Part model, mm, in its own coordinate system. Coordinates: 2 decimals unless noted, no trailing zeros. Loops run counter-clockwise (first coordinate to the right, second up) from the corner with the lowest first, then second, coordinate; pieces in that order, holes last. Notation, with made-up numbers: (33.5, 73) - (91.5, 73) arc R5 ccw to (91.5, 82) - close; hole circle Ø9 at (18, 17). An arc over 180 degrees is marked (long way). Use a Markdown table: item, result. Add a question column.
1) Probe probe 1 along Z at (x, y) = (110, -2.5); probe 2 along Z at (x, y) = (25.4, -0.8); probe 3 along Z at (x, y) = (61, -2.2). List the from-to ranges inside material, lowest first. Write a range as [from, to].
2) Band-saw the part on C-C (x = 109). Give the cut face in (y, z) (3 decimals), plus the area to 3 significant figures.
3) Band-saw the part on B-B (y = -1.05). Give the number of separate pieces and of enclosed holes in the cut face, plus the area to 3 significant figures.
4) Pull direction Z, two halves, no side cores. Call faces 1 (the face through (141.064, -1.565, 99.69)), 2 (the face through (0, -2, 51)), 3 (the face through (87.24, -1.57, 96.22)): +Z half, -Z half, draft (parallel to the pull), parting line (faces both ways), or undercut.
5) Drop flat-ended pins along their axis: P1, Ø8.5, axis at x = 136.525, z = 38.1, coming from the +Y side; P2, Ø6.5, axis at x = 92.075, z = 76.2, coming from the -Y side. Give the stop position or say it passes through.
6) Band-saw the part on D-D (z = 38.1). Give the cut face in (x, y) (1 decimal), plus the area to 3 significant figures.
7) Band-saw the part on A-A (z = 88.9). Give the cut face in (x, y) (1 decimal).
from build123d import *

# Parameters (mm, degrees)
F0_R     = 3.2385
F0_R_2   = 2.54
F0_R_3   = 4.191
F0_R_4   = 14.2875
F0_R_5   = 4.7625
F1_DEPTH = 3.175


with BuildPart() as f1:
    # F0 (on Front) → F1 (new body)
    with BuildSketch(Plane.XZ):
        with BuildLine():
            ThreePointArc((0, 6.35), (1.859872, 1.859872), (6.35, 0))
            Line((6.35, 0), (136.525, 0))
            ThreePointArc((136.525, 0), (141.015128, 1.859872), (142.875, 6.35))
            Line((142.875, 6.35), (142.875, 95.25))
            ThreePointArc((142.875, 95.25), (141.015128, 99.740128), (136.525, 101.6))
            Line((136.525, 101.6), (6.35, 101.6))
            ThreePointArc((6.35, 101.6), (1.859872, 99.740128), (0, 95.25))
            Line((0, 95.25), (0, 6.35))
        make_face()
        with Locations((33.3502, 6.35)):
            Circle(F0_R, mode=Mode.SUBTRACT)
        with Locations((6.35, 12.7)):
            Circle(F0_R, mode=Mode.SUBTRACT)
        with Locations((58.7502, 6.35)):
            Circle(F0_R, mode=Mode.SUBTRACT)
        with Locations((25.4, 25.4)):
            Circle(F0_R_2, mode=Mode.SUBTRACT)
        with Locations((6.35, 38.1)):
            Circle(F0_R, mode=Mode.SUBTRACT)
        with Locations((84.1502, 6.35)):
            Circle(F0_R, mode=Mode.SUBTRACT)
        with Locations((109.5502, 6.35)):
            Circle(F0_R, mode=Mode.SUBTRACT)
        with Locations((136.525, 12.7)):
            Circle(F0_R, mode=Mode.SUBTRACT)
        with Locations((92.075, 25.4)):
            Circle(F0_R_3, mode=Mode.SUBTRACT)
        with Locations((117.475, 25.4)):
            Circle(F0_R_2, mode=Mode.SUBTRACT)
        with Locations((136.525, 38.1)):
            Circle(F0_R, mode=Mode.SUBTRACT)
        with Locations((6.35, 63.5)):
            Circle(F0_R, mode=Mode.SUBTRACT)
        with Locations((51.3842, 50.8)):
            Circle(F0_R_4, mode=Mode.SUBTRACT)
        with Locations((25.4, 76.2)):
            Circle(F0_R_2, mode=Mode.SUBTRACT)
        with Locations((6.35, 88.9)):
            Circle(F0_R, mode=Mode.SUBTRACT)
        with Locations((33.3502, 95.25)):
            Circle(F0_R, mode=Mode.SUBTRACT)
        with Locations((58.7502, 95.25)):
            Circle(F0_R, mode=Mode.SUBTRACT)
        with Locations((92.075, 50.8)):
            Circle(F0_R_5, mode=Mode.SUBTRACT)
        with Locations((136.525, 63.5)):
            Circle(F0_R, mode=Mode.SUBTRACT)
        with Locations((92.075, 76.2)):
            Circle(F0_R_3, mode=Mode.SUBTRACT)
        with Locations((84.1502, 95.25)):
            Circle(F0_R, mode=Mode.SUBTRACT)
        with Locations((117.475, 76.2)):
            Circle(F0_R_2, mode=Mode.SUBTRACT)
        with Locations((109.5502, 95.25)):
            Circle(F0_R, mode=Mode.SUBTRACT)
        with Locations((136.525, 88.9)):
            Circle(F0_R, mode=Mode.SUBTRACT)
    extrude(amount=F1_DEPTH)


solid = f1.part
Answer block:
| question | item | result |
|---|---|---|
| 1 | probe 1 | [0, 3.14], [9.56, 92.04], [98.46, 101.6] |
| 1 | probe 2 | [0, 22.86], [27.94, 73.66], [78.74, 101.6] |
| 1 | probe 3 | [0, 4.02], [8.68, 40.23], [61.37, 92.92], [97.58, 101.6] |
| 2 | outline | (-3.175, 0) - (0, 0) - (0, 3.159) - (-3.175, 3.159) - close; (-3.175, 9.541) - (0, 9.541) - (0, 92.059) - (-3.175, 92.059) - close; (-3.175, 98.441) - (0, 98.441) - (0, 101.6) - (-3.175, 101.6) - close |
| 2 | area | 282 mm2 |
| 3 | separate pieces | 1 |
| 3 | enclosed holes | 24 |
| 3 | area | 13,100 mm2 |
| 4 | face 1 | +Z half |
| 4 | face 2 | draft |
| 4 | face 3 | undercut |
| 5 | P1 | y = 0 |
| 5 | P2 | through |
| 6 | outline | (0, -3.2) - (3.1, -3.2) - (3.1, 0) - (0, 0) - close; (9.6, -3.2) - (44.8, -3.2) - (44.8, 0) - (9.6, 0) - close; (57.9, -3.2) - (133.3, -3.2) - (133.3, 0) - (57.9, 0) - close; (139.8, -3.2) - (142.9, -3.2) - (142.9, 0) - (139.8, 0) - close |
| 6 | area | 371 mm2 |
| 7 | outline | (0, -3.2) - (3.1, -3.2) - (3.1, 0) - (0, 0) - close; (9.6, -3.2) - (133.3, -3.2) - (133.3, 0) - (9.6, 0) - close; (139.8, -3.2) - (142.9, -3.2) - (142.9, 0) - (139.8, 0) - close |
